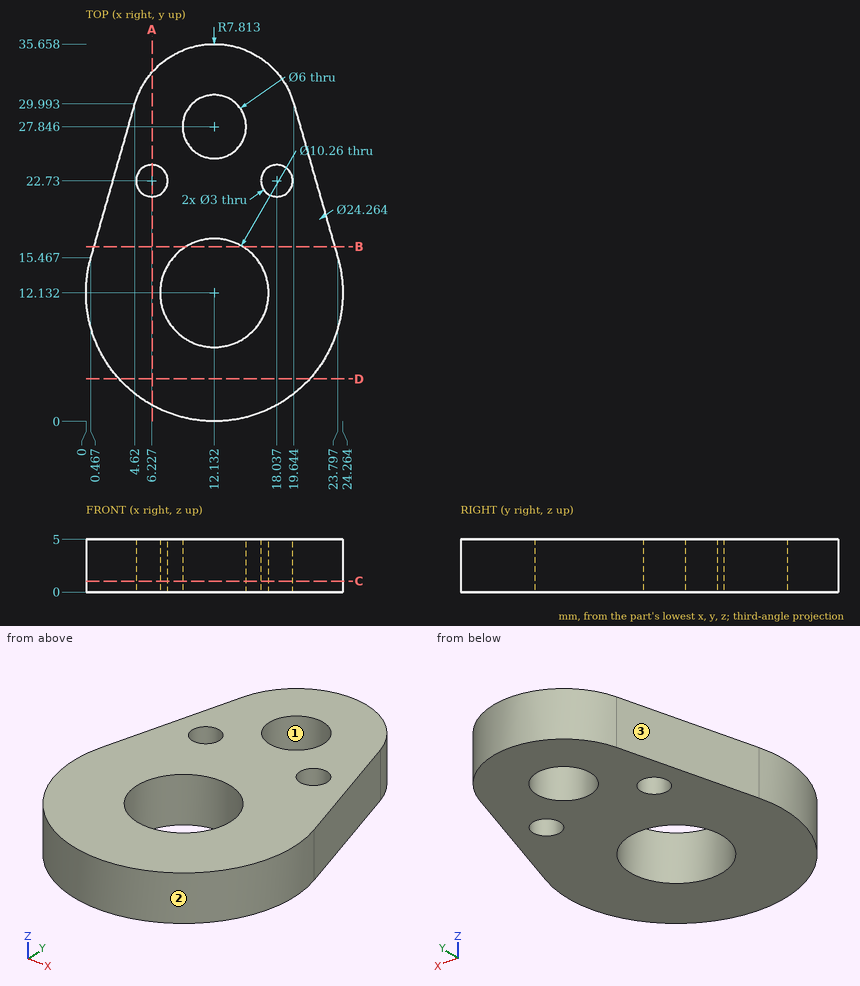
Input: dimensioned drawing with shaded views. Units: mm. Origin: part minimum x, y, z. Give positions to 0.01 mm unless a question says otherwise; leave off trailing zeros. Loops run counter-clockwise (first coordinate to the right, second up) from the corner with the lowest first, then second, coordinate; pieces in that order, holes last. Notation, with made-up numbers: (82, 89) -> (132, 89) arc R16 ccw to (132, 112) -> close; hole circle Ø11 at (21.25, -14). An arc over 180 degrees is marked (long way). Use a Markdown table: item, result. Add a question column.
1) Section query B-B, the plane y = 16.5. Return the cut outline in (x, z).
2) First-contact query: pin 1 (5 mm diameter, centred on x = 6.23, y = 22.73, fed in from +Z); pin 2 (1.5 mm diameter, centred on x = 11, y = 9.5, fed in from +Z); pin 3 (1.5 mm diameter, centred on x = 7, z = 4.5, fed in from +Y) (1 decimal). Flat tips, straight axial feed; report the tip coordinate or a pass-through.
3) Line query: line 1 along X through (y, z) = (16.5, 1.7) (1 decimal); line 2 along Y through (x, z) = (10, 4.1) (1 decimal); line 3 along X through (y, z) = (26.5, 3.5). Output: solid intervals per line, ascending. Write a range as [from, to].
4) Pull-direction query (Y, two-part tool) for the marked faces 1, 2 and 3; classes: +Y half, -Y half, draft (parallel to the pull), parting line (faces both ways), or undercut.
5) Section query D-D, the plane y = 4. Return the cut outline in (x, z) (1 decimal).
6) Section query C-C, the plane z = 1.05. Return the cut outline in (x, y) (1 decimal).
7) Section query A-A, the plane x = 6.25. Return the cut outline in (y, z), then the cut area to 3 significant figures.
Numbers:
| question | item | result |
|---|---|---|
| 1 | outline | (0.76, 0) -> (9.44, 0) -> (9.44, 5) -> (0.76, 5) -> close; (14.82, 0) -> (23.5, 0) -> (23.5, 5) -> (14.82, 5) -> close |
| 2 | pin 1 | stops at z = 5 |
| 2 | pin 2 | passes through |
| 2 | pin 3 | stops at y = 34.3 |
| 3 | line 1 | x = [0.8, 9.4], [14.8, 23.5] |
| 3 | line 2 | y = [0.2, 7.5], [16.8, 25.7], [30, 35.4] |
| 3 | line 3 | x = [3.62, 9.45], [14.81, 20.64] |
| 4 | face 1 | undercut |
| 4 | face 2 | parting line |
| 4 | face 3 | +Y half |
| 5 | outline | (3.1, 0) -> (21.1, 0) -> (21.1, 5) -> (3.1, 5) -> close |
| 6 | outline | (0.5, 15.5) arc R12.1 ccw (long way) to (23.8, 15.5) -> (19.6, 30) arc R7.8 ccw to (4.6, 30) -> close; hole circle Ø3 at (6.2, 22.7); hole circle Ø10.3 at (12.1, 12.1); hole circle Ø6 at (12.1, 27.8); hole circle Ø3 at (18, 22.7) |
| 7 | outline | (1.52, 0) -> (21.23, 0) -> (21.23, 5) -> (1.52, 5) -> close; (24.23, 0) -> (32.99, 0) -> (32.99, 5) -> (24.23, 5) -> close |
| 7 | area | 142 mm2 |
